```python
from build123d import *

# Parameters (mm, degrees)
F0_W     = 38.1
F0_H     = 12.7
F1_DEPTH = 25.4
F3_DEPTH = 12.7


with BuildPart() as f1:
    # F0 (on Front) → F1 (new body)
    with BuildSketch(Plane.XZ):
        with Locations((19.05, 6.35)):
            Rectangle(F0_W, F0_H)
    extrude(amount=F1_DEPTH)

    # F2 (on face) → F3 (join)
    with BuildSketch(Plane.XY.offset(12.7)):
        Polygon((6.35, -25.4), (31.75, 0), (0, 0), (0, -25.4), align=None)
        Polygon((38.1, -12.7), (25.4, -25.4), (38.1, -25.4), align=None)
    extrude(amount=F3_DEPTH)


solid = f1.part
```
Geometry: final body of the model. Coordinates: model frame, mm. A direction names the side the tool comes from. Round coordinates to 2 decimals unless told otherwise and drop trailing zeros. Loops run counter-clockwise (first coordinate to the right, second up) from the corner with the lowest first, then second, coordinate; pieces in that order, holes last. Notation, with made-up numbers: (-20, -37) -> (1, -37) arc R31 cw to (1, -4) -> close; hole circle Ø5 at (-30.75, 22). An arc over 180 degrees is marked (long way). Write each question's results on one line, items separated by ' | '.
Item 1: Cut plane B-B on y = -18.5. Return the cut outline in (x, z).
Answers below:
outline: (0, 0) -> (38.1, 0) -> (38.1, 25.4) -> (32.3, 25.4) -> (32.3, 12.7) -> (13.25, 12.7) -> (13.25, 25.4) -> (0, 25.4) -> close
Item 2: Pull-direction query (Y, two-part tool) for faces 3 (the face through (19, 0, 13)), 4 (the face through (19, -25.4, 10)), 5 (the face through (26, -15, 12.7)); classes: pulls with the +Y half, pulls with the -Y half, needs draft (parallel to the pull), parting line crosses it, or undercut.
Answers below:
face 3: pulls with the +Y half | face 4: pulls with the -Y half | face 5: undercut
Item 3: Cut plane D-D on y = -4. Return the cut outline in (x, z).
Answers below:
outline: (0, 0) -> (38.1, 0) -> (38.1, 12.7) -> (27.75, 12.7) -> (27.75, 25.4) -> (0, 25.4) -> close
Item 4: Set-up query: faces 1 (the face through (34, -22, 25.4)), 2 (the face through (18.87, -12.88, 18.96)). Return all of +Z, -Z, +X, -X, +Y, -Y with unobstructed straight access to the full face (end or side cutting, diameter ignored); none if empty.
Answers below:
face 1: +Z, +X, -X, +Y, -Y | face 2: +Z
Item 5: Cut plane C-C on x = 30. Return the cut outline in (y, z), and give its area (3 significant figures).
Answers below:
outline: (-25.4, 0) -> (0, 0) -> (0, 25.4) -> (-1.75, 25.4) -> (-1.75, 12.7) -> (-20.8, 12.7) -> (-20.8, 25.4) -> (-25.4, 25.4) -> close | area: 403 mm²
Item 6: Cut plane A-A on z = 22.5. Return the cut outline in (x, y).
Answers below:
outline: (0, -25.4) -> (6.35, -25.4) -> (31.75, 0) -> (0, 0) -> close; (25.4, -25.4) -> (38.1, -25.4) -> (38.1, -12.7) -> close
Item 7: Line query: probe 1 along Z at (x, y) = (28, -9.75); probe 2 along Y at (x, z) = (30, 17.75); probe 3 along X at (y, z) = (-20.75, 21.75). Output: solid intervals per line, ascending. Write a range as [from, to].
Answers below:
probe 1: z = [0, 12.7] | probe 2: y = [-25.4, -20.8], [-1.75, 0] | probe 3: x = [0, 11], [30.05, 38.1]
